from build123d import *

# Parameters (mm, degrees)
ESQUISSE1_R                  = 8.5
BOSS_EXTRU_1_DEPTH           = 18.4
ESQUISSE2_W                  = 6.4
ESQUISSE2_H                  = 3.4
BOSS_EXTRU_2_DEPTH           = 2.6
ESQUISSE3_W                  = 0.5
ESQUISSE3_H                  = 0.5
BOSS_EXTRU_3_DEPTH           = 3
CHANFREIN1_SIZE              = 0.1
ESQUISSE4_W                  = 12
ESQUISSE4_H                  = 4
ENL_V_MAT_EXTRU_1_DEPTH      = 27.453922204
ESQUISSE5_R                  = 1
ENL_V_MAT_EXTRU_2_DEPTH      = 5
ENL_V_MAT_EXTRU_3_DEPTH      = 12.5
ENL_V_MAT_EXTRU_3_DEPTH_BACK = 0.5
ESQUISSE6_R                  = 6.493106385
ESQUISSE7_R                  = 2.5
BOSS_EXTRU_4_DEPTH           = 5
ESQUISSE8_R                  = 6
BOSS_EXTRU_5_DEPTH           = 0.5
ESQUISSE10_R                 = 1
ENL_V_MAT_EXTRU_4_DEPTH      = 10


with BuildPart() as part:
    # Esquisse1 → Boss.-Extru.1 (new body)
    with BuildSketch(Plane.XY):
        Circle(ESQUISSE1_R)
    extrude(amount=BOSS_EXTRU_1_DEPTH)

    # Esquisse2 → Boss.-Extru.2 (add)
    with BuildSketch(Plane(origin=(0, 0, 0), x_dir=(-1, 0, 0), z_dir=(0, 0, -1))):
        with Locations((0, -4.3)):
            Rectangle(ESQUISSE2_W, ESQUISSE2_H)
    extrude(amount=BOSS_EXTRU_2_DEPTH)

    # Esquisse3 → Boss.-Extru.3 (add)
    with BuildSketch(Plane(origin=(0, 0, -2.6), x_dir=(-1, 0, 0), z_dir=(0, 0, -1))):
        with Locations((-1.23, -3.415159268)):
            Rectangle(ESQUISSE3_W, ESQUISSE3_H)
        with Locations((-2.5, -3.415159268)):
            Rectangle(ESQUISSE3_W, ESQUISSE3_H)
        with Locations((0.04, -3.415159268)):
            Rectangle(ESQUISSE3_W, ESQUISSE3_H)
        with Locations((1.31, -3.415159268)):
            Rectangle(ESQUISSE3_W, ESQUISSE3_H)
        with Locations((2.58, -3.415159268)):
            Rectangle(ESQUISSE3_W, ESQUISSE3_H)
        with Locations((-2.5, -4.685159268)):
            Rectangle(ESQUISSE3_W, ESQUISSE3_H)
        with Locations((-1.23, -4.685159268)):
            Rectangle(ESQUISSE3_W, ESQUISSE3_H)
        with Locations((0.04, -4.685159268)):
            Rectangle(ESQUISSE3_W, ESQUISSE3_H)
        with Locations((1.31, -4.685159268)):
            Rectangle(ESQUISSE3_W, ESQUISSE3_H)
        with Locations((2.58, -4.685159268)):
            Rectangle(ESQUISSE3_W, ESQUISSE3_H)
    extrude(amount=BOSS_EXTRU_3_DEPTH)

    # Chanfrein1
    chanfrein1_edges = [part.edges().sort_by_distance(p)[0] for p in [
        (-1.06, -4.685159268, -5.6),
        (-1.31, -4.935159268, -5.6),
        (-1.56, -4.685159268, -5.6),
        (-1.31, -4.435159268, -5.6),
        (-2.33, -4.685159268, -5.6),
        (-2.58, -4.935159268, -5.6),
        (-2.83, -4.685159268, -5.6),
        (-2.58, -4.435159268, -5.6),
        (2.75, -3.415159268, -5.6),
        (2.5, -3.665159268, -5.6),
        (2.25, -3.415159268, -5.6),
        (2.5, -3.165159268, -5.6),
        (1.48, -3.415159268, -5.6),
        (1.23, -3.665159268, -5.6),
        (0.98, -3.415159268, -5.6),
        (1.23, -3.165159268, -5.6),
        (0.21, -3.415159268, -5.6),
        (-0.04, -3.665159268, -5.6),
        (-0.29, -3.415159268, -5.6),
        (-0.04, -3.165159268, -5.6),
        (-1.06, -3.415159268, -5.6),
        (-1.31, -3.665159268, -5.6),
        (-1.56, -3.415159268, -5.6),
        (-1.31, -3.165159268, -5.6),
        (-2.33, -3.415159268, -5.6),
        (-2.58, -3.665159268, -5.6),
        (-2.83, -3.415159268, -5.6),
        (-2.58, -3.165159268, -5.6),
        (2.75, -4.685159268, -5.6),
        (2.5, -4.935159268, -5.6),
        (2.25, -4.685159268, -5.6),
        (2.5, -4.435159268, -5.6),
        (1.48, -4.685159268, -5.6),
        (1.23, -4.935159268, -5.6),
        (0.98, -4.685159268, -5.6),
        (1.23, -4.435159268, -5.6),
        (0.21, -4.685159268, -5.6),
        (-0.04, -4.935159268, -5.6),
        (-0.29, -4.685159268, -5.6),
        (-0.04, -4.435159268, -5.6),
    ]]
    chamfer(chanfrein1_edges, length=CHANFREIN1_SIZE)

    # Esquisse4 → Enlèv. mat.-Extru.1 (cut, through all)
    with BuildSketch(Plane(origin=(8.5, 0, 0), x_dir=(0, 0, -1), z_dir=(1, 0, 0))):
        with Locations((-8, -6.5)):
            Rectangle(ESQUISSE4_W, ESQUISSE4_H)
    extrude(amount=-ENL_V_MAT_EXTRU_1_DEPTH, mode=Mode.SUBTRACT)

    # Esquisse5 → Enlèv. mat.-Extru.2 (cut)
    with BuildSketch(Plane.XY.offset(18.4)):
        with Locations((-6, 0)):
            Circle(ESQUISSE5_R)
        with Locations((6, 0)):
            Circle(ESQUISSE5_R)
    extrude(amount=-ENL_V_MAT_EXTRU_2_DEPTH, mode=Mode.SUBTRACT)

    # Esquisse6 → Enlèv. mat.-Extru.3 (cut, two sides: drawn at the far end of the back side and taken through both)
    with BuildSketch(Plane.XY.offset(2).offset(-ENL_V_MAT_EXTRU_3_DEPTH_BACK)):
        Circle(ESQUISSE6_R)
    extrude(amount=ENL_V_MAT_EXTRU_3_DEPTH + ENL_V_MAT_EXTRU_3_DEPTH_BACK, mode=Mode.SUBTRACT)

    # Esquisse7 → Boss.-Extru.4 (add)
    with BuildSketch(Plane.XY.offset(1.5)):
        Circle(ESQUISSE7_R)
    extrude(amount=BOSS_EXTRU_4_DEPTH)

    # Esquisse8 → Boss.-Extru.5 (add)
    with BuildSketch(Plane.XY.offset(6.5)):
        Circle(ESQUISSE8_R)
    extrude(amount=BOSS_EXTRU_5_DEPTH)

    # Esquisse10 → Enlèv. mat.-Extru.4 (cut)
    with BuildSketch(Plane.XY.offset(18.4)):
        Circle(ESQUISSE10_R)
    extrude(amount=-ENL_V_MAT_EXTRU_4_DEPTH, mode=Mode.SUBTRACT)


solid = part.part
Verification items for the finished model (mm, model axes). A direction names the side the tool comes from. Give positions to 0.01 mm unless a question says otherwise; leave off trailing zeros. Write each loop counter-clockwise with the first axis right and the second up, starting at its lowest first coordinate (ties: lowest second). Pieces come first, ordered by that corner, then holes. Notation, with made-up numbers: M 12.5,42 L 56.5,42 A32 cw 56.5,71 Z; hole C -32.5,-25.75 d9. An arc over 180 degrees is marked long. Put each result on its own line as item: value. Start each with the question number.
1. Go/stop test with flat-tipped pins: pin 1 Ø0.6 at (y, z) = (-3.5, -4.5) entering from -X; pin 2 Ø6 at (y, z) = (-4, -2) entering from -X; pin 3 Ø8 at (x, z) = (4.5, 7.5) entering from +Y; pin 4 Ø2.5 at (x, y) = (6, 0) entering from +Z. Record where each tip stops, or that it passes through.
2. Section check A-A (y = 0). Record the cut outline in (x, z), and give its area (3 significant figures).
3. Section check B-B (y = 5). Record the cut outline in (x, z), and give its area (3 significant figures).
4. Draft check along Z on faces 5 (the face through (-6, -4.5, 8)), 6 (the face through (-3.2, -4, -1)), 7 (the face through (2, 0, 18.4)). Enter one of: +Z half, -Z half, draft (parallel to the pull), parting line (faces both ways), or undercut.
5. Set-up check for faces 1 (the face through (3.2, -4, -1)), 2 (the face through (0, -7, 14)), 3 (the face through (-0.845, 6.438, 7.909)), 4 (the face through (0, -1, 16)): record each of +Z, -Z, +X, -X, +Y, -Y from which the full face is reachable in a straight line by a thin tool's end or side.
6. Section check D-D (z = 12). Record the cut outline in (x, y).
7. Section check C-C (x = -4). Record the cut outline in (y, z), and give its area (3 significant figures).
8. Scan lines: line 1 along Z through (x, y) = (-3.25, -3.5); line 2 along Z through (x, y) = (-3.75, 5.25); line 3 along Z through (x, y) = (-5.5, -0.75). Record each from-to range of solid material in increasing order. Write a range as [from, to].
Answer list:
1. pin 1: x = -2.83
1. pin 2: x = -8.31
1. pin 3: y = 8.49
1. pin 4: z = 18.4
2. outline: M -8.5,0 L 8.5,0 L 8.5,18.4 L 7,18.4 L 7,13.4 L 6.49,13.4 L 6.49,1.5 L 2.5,1.5 L 2.5,6.5 L 6,6.5 L 6,7 L -6,7 L -6,6.5 L -2.5,6.5 L -2.5,1.5 L -6.49,1.5 L -6.49,13.4 L -7,13.4 L -7,18.4 L -8.5,18.4 Z; M -5,14.5 L -1,14.5 L -1,18.4 L -5,18.4 Z; M 1,14.5 L 5,14.5 L 5,18.4 L 1,18.4 Z
2. area: 150 mm2
3. outline: M -6.87,0 L 6.87,0 L 6.87,18.4 L -6.87,18.4 Z; M -3.32,6.5 L 3.32,6.5 L 3.32,7 L -3.32,7 Z; hole M -4.14,1.5 L 4.14,1.5 L 4.14,14.5 L -4.14,14.5 Z
3. area: 149 mm2
4. face 5: undercut
4. face 6: draft
4. face 7: +Z half
5. face 1: -Z, +X, +Y, -Y
5. face 2: +X, -X, -Y
5. face 3: none
5. face 4: +Z
6. outline: M -7.21,-4.5 L -4.68,-4.5 A6.49 cw long 4.68,-4.5 L 7.21,-4.5 A8.5 ccw long Z
7. outline: M -7.5,0 L 7.5,0 L 7.5,18.4 L -7.5,18.4 L -7.5,14 L -5.11,14 L -5.11,14.5 L 5.11,14.5 L 5.11,1.5 L -5.11,1.5 L -5.11,2 L -7.5,2 Z; M -4.47,6.5 L 4.47,6.5 L 4.47,7 L -4.47,7 Z
7. area: 119 mm2
8. line 1: [0, 1.5], [6.5, 7], [14.5, 18.4]
8. line 2: [0, 1.5], [14.5, 18.4]
8. line 3: [0, 1.5], [6.5, 7]
